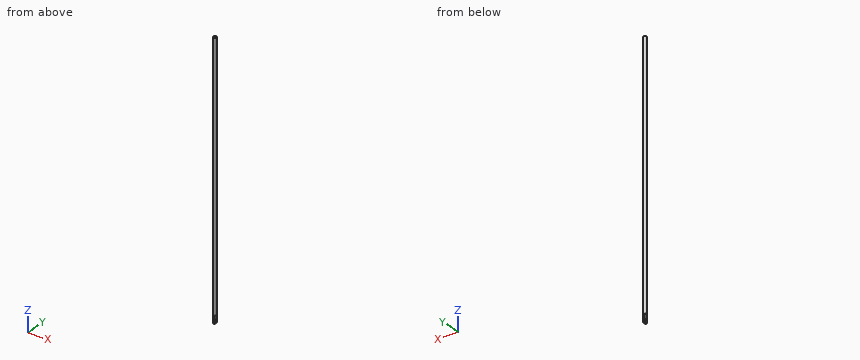
```python
from build123d import *

# Parameters (mm, degrees)
SKETCH1_R                      = 1.5875
BOSS_EXTRUDE1_DEPTH            = 254
CUT_EXTRUDE1_DEPTH             = 255.009921681
CUT_EXTRUDE1_DEPTH_BACK        = 255.009921681
SKETCH2_W                      = 0.8255
SKETCH2_H                      = 7.62
CUT_EXTRUDE2_REACH             = 256.01
SKETCH3_R                      = 0.762
CUT_EXTRUDE2_DIRECTION_2_REACH = 256.01


with BuildPart() as part:
    # Sketch1 → Boss-Extrude1 (new body)
    with BuildSketch(Plane.XY):
        Circle(SKETCH1_R)
    extrude(amount=BOSS_EXTRUDE1_DEPTH)

    # Sketch2 → Cut-Extrude1 (cut, two sides: drawn at the far end of the back side and taken through both)
    with BuildSketch(Plane(origin=(0, 0, 0), x_dir=(1, 0, 0), z_dir=(0, 1, 0)).offset(-CUT_EXTRUDE1_DEPTH_BACK)):
        with Locations((1.17475, -3.81)):
            Rectangle(SKETCH2_W, SKETCH2_H)
        with Locations((-1.17475, -3.81)):
            Rectangle(SKETCH2_W, SKETCH2_H)
    extrude(amount=CUT_EXTRUDE1_DEPTH + CUT_EXTRUDE1_DEPTH_BACK, mode=Mode.SUBTRACT)

    # Sketch3 → Cut-Extrude2 (cut, up to next)
    with BuildSketch(Plane(origin=(0, 0, 0), x_dir=(0, 0, -1), z_dir=(1, 0, 0)), mode=Mode.PRIVATE) as cut_extrude2_sk1:
        with Locations(Location((-2.54, 0, 0), (0, 0, 180))):
            Circle(SKETCH3_R)
    cut_extrude2_tool1 = extrude(cut_extrude2_sk1.sketch, amount=-CUT_EXTRUDE2_REACH, mode=Mode.PRIVATE) & part.part
    add(cut_extrude2_tool1.solids().sort_by_distance((0, 0, 2.54))[0], mode=Mode.SUBTRACT)

    # Sketch3 → Cut-Extrude2 direction 2 (cut, up to next)
    with BuildSketch(Plane(origin=(0, 0, 0), x_dir=(0, 0, -1), z_dir=(1, 0, 0)), mode=Mode.PRIVATE) as cut_extrude2_direction_2_sk1:
        with Locations(Location((-2.54, 0, 0), (0, 0, 180))):
            Circle(SKETCH3_R)
    cut_extrude2_direction_2_tool1 = extrude(cut_extrude2_direction_2_sk1.sketch, amount=CUT_EXTRUDE2_DIRECTION_2_REACH, mode=Mode.PRIVATE) & part.part
    add(cut_extrude2_direction_2_tool1.solids().sort_by_distance((0, 0, 2.54))[0], mode=Mode.SUBTRACT)


solid = part.part
```
Check sheet for the modelled part. Datum: model origin and axes. Units: mm. Coordinates: 2 decimals unless noted, no trailing zeros. Write each loop counter-clockwise with the first axis right and the second up, starting at its lowest first coordinate (ties: lowest second). Pieces come first, ordered by that corner, then holes. Notation, with made-up numbers: (-24, -26) - (-11, -26) arc R20 cw to (-11, -13) - close; hole circle Ø4 at (58, 9.25). An arc over 180 degrees is marked (long way). One line per question, with ' | ' between items.
Item 1: Gauge pin test, flat end, axial feed: P1, Ø1.5, axis at x = -1, z = 109, coming from the +Y side. Record the tip position at first contact, or that the pin passes through.
Determined:
P1: stops at y = 1.57
Item 2: Thickness scan on line 1 (Y direction, x = 0.2, z = 2.54); line 2 (Z direction, x = -1.15, y = 0.6); line 3 (Y direction, x = -0.25, z = 177). Record the ranges inside material, lowest first. Write a range as [from, to].
Determined:
line 1: y = [-1.57, -0.76], [0.76, 1.57] | line 2: z = [7.62, 254] | line 3: y = [-1.57, 1.57]
Item 3: Sectioned sample at A-A on z = 18.5. Record the boundary of the cut face in (x, y) (1 decimal), plus the area to 3 significant figures.
Determined:
outline: circle Ø3.2 at (0, 0) | area: 7.92 mm2
